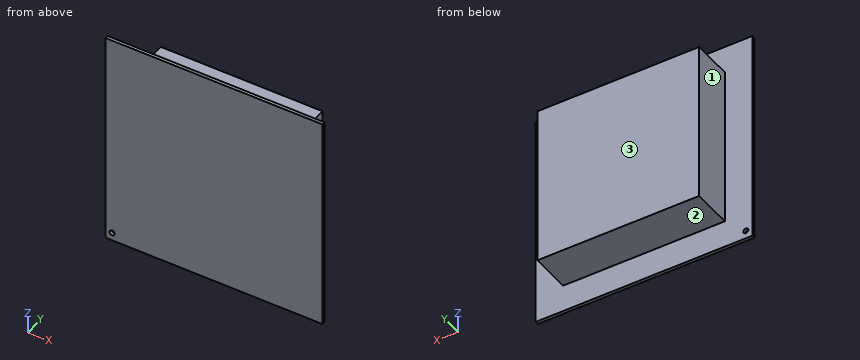
from build123d import *

# Parameters (mm, degrees)
SKETCH1_W                 = 170.18
SKETCH1_H                 = 170.18
BOSS_EXTRUDE1_DEPTH       = 2.54
SKETCH2_W                 = 127
SKETCH2_H                 = 127
BOSS_EXTRUDE2_DEPTH       = 31.75
F_4_0MM_DOWEL_HOLE1_D     = 4
F_4_0MM_DOWEL_HOLE1_DEPTH = 12.7
F_4_0MM_DOWEL_HOLE1_TIP   = 1.201721238


with BuildPart() as part:
    # Sketch1 → Boss-Extrude1 (new body)
    with BuildSketch(Plane(origin=(0, 0, 0), x_dir=(1, 0, 0), z_dir=(0, 1, 0))):
        Rectangle(SKETCH1_W, SKETCH1_H)
    extrude(amount=BOSS_EXTRUDE1_DEPTH)

    # Sketch2 → Boss-Extrude2 (add)
    with BuildSketch(Plane(origin=(0, 2.54, 0), x_dir=(1, 0, 0), z_dir=(0, 1, 0))):
        Rectangle(SKETCH2_W, SKETCH2_H)
    extrude(amount=BOSS_EXTRUDE2_DEPTH)

    # Ø4.0mm Dowel Hole1
    with Locations(Plane(origin=(0, 2.54, 0), x_dir=(1, 0, 0), z_dir=(0, 1, 0))):
        with Locations((-80.01, 78.74)):
            Hole(F_4_0MM_DOWEL_HOLE1_D / 2, depth=F_4_0MM_DOWEL_HOLE1_DEPTH)
            with Locations((0, 0, -(F_4_0MM_DOWEL_HOLE1_DEPTH + F_4_0MM_DOWEL_HOLE1_TIP / 2))):  # 118° drill point
                Cone(0, F_4_0MM_DOWEL_HOLE1_D / 2, F_4_0MM_DOWEL_HOLE1_TIP, mode=Mode.SUBTRACT)


solid = part.part
Build history of the part. All positions in model axes, mm. Face numbers are marked on the shaded views. A direction names the side the tool comes from. Coordinates: 2 decimals unless noted, no trailing zeros. Write each loop counter-clockwise with the first axis right and the second up, starting at its lowest first coordinate (ties: lowest second). Pieces come first, ordered by that corner, then holes. Notation, with made-up numbers: (61, 50.25) -> (89, 50.25) arc R34 ccw to (89, 81.25) -> close; hole circle Ø3 at (39, 87). An arc over 180 degrees is marked (long way). Use CSV: the item, a comma, the result in double quotes. Start each with the question number.
Q1. Drill centre lines: probe 1 along Z at (x, y) = (-80, 1); probe 2 along X at (y, z) = (1.45, -78.74); probe 3 along Z at (x, y) = (54, 17). Where is each one in solid material? Low to high.
Q2. Flat gauge pins, fed straight in: pin 1 Ø5 at (x, y) = (56, 25.5) entering from -Z; pin 2 Ø8 at (y, z) = (26, 66.5) entering from -X; pin 3 Ø8 at (y, z) = (9, 22.5) entering from +X. Where does each tip first touch, or does it go through?
Q3. Cut at A-A, the plane z = -78.74. List the corners of the cut face in (x, y), then the cut area to 3 significant figures.
Q4. Cut at D-D, the plane z = 6. List the corners of the cut face in (x, y), then the cut area to 3 significant figures.
Q5. Cut at B-B, the plane x = -80.01. List the corners of the cut face in (y, z).
Q6. Cut at C-C, the plane x = 23. List the corners of the cut face in (y, z), then the cut area to 3 significant figures.
Q7. 3-axis set-ups, long thin cutter, end or side, ignore diameter. For the marked faces 1, 2 and 3: which of +Z, -Z, +X, -X, +Y, -Y reach the whole face in a straight line?
Checked values:
1,probe 1,"z = -85.09 to -80.74, -76.74 to 85.09"
1,probe 2,"x = -85.09 to -82.01, -78.01 to 85.09"
1,probe 3,"z = -63.5 to 63.5"
2,pin 1,"stops at z = -63.5"
2,pin 2,"stops at x = -63.5"
2,pin 3,"stops at x = 63.5"
3,outline,"(-85.09, 0) -> (-82.01, 0) -> (-82.01, 2.54) -> (-85.09, 2.54) -> close; (-78.01, 0) -> (85.09, 0) -> (85.09, 2.54) -> (-78.01, 2.54) -> close"
3,area,"422 mm²"
4,outline,"(-85.09, 0) -> (85.09, 0) -> (85.09, 2.54) -> (63.5, 2.54) -> (63.5, 34.29) -> (-63.5, 34.29) -> (-63.5, 2.54) -> (-85.09, 2.54) -> close"
4,area,"4,460 mm²"
5,outline,"(0, -85.09) -> (2.54, -85.09) -> (2.54, -80.74) -> (0, -80.74) -> close; (0, -76.74) -> (2.54, -76.74) -> (2.54, 85.09) -> (0, 85.09) -> close"
6,outline,"(0, -85.09) -> (2.54, -85.09) -> (2.54, -63.5) -> (34.29, -63.5) -> (34.29, 63.5) -> (2.54, 63.5) -> (2.54, 85.09) -> (0, 85.09) -> close"
6,area,"4,460 mm²"
7,face 1,"+Z, -Z, -X, +Y"
7,face 2,"-Z, +X, -X, +Y"
7,face 3,"+Z, -Z, +X, -X, +Y"
